CAD build for the part. Positions are in the model's coordinates, mm. Face numbers are marked on the shaded views. A direction names the side the tool comes from. Give positions to 0.01 mm unless a question says otherwise; leave off trailing zeros. Write each loop counter-clockwise with the first axis right and the second up, starting at its lowest first coordinate (ties: lowest second). Pieces come first, ordered by that corner, then holes. Notation, with made-up numbers: (-2.5, -17) - (11.5, -17) arc R31 cw to (11.5, 18) - close; hole circle Ø7 at (-26.5, 53.25). An arc over 180 degrees is marked (long way). Answer as a JSON object with one key per item and string values.
from build123d import *

# Parameters (mm, degrees)
CROQUIS1_W              = 202
CROQUIS1_H              = 100
SALIENTE_EXTRUIR1_DEPTH = 1.5
CROQUIS2_R              = 1.6
CORTAR_EXTRUIR1_DEPTH   = 1.5
CROQUIS3_W              = 12
CROQUIS3_H              = 100
CROQUIS3_R              = 1.6
SALIENTE_EXTRUIR2_DEPTH = 6
CROQUIS4_W              = 47
CROQUIS4_H              = 28
CROQUIS4_W_2            = 76
SALIENTE_EXTRUIR3_DEPTH = 1.5
REDONDEO1_R             = 10
REDONDEO2_R             = 10
CROQUIS5_R              = 3
CORTAR_EXTRUIR2_DEPTH   = 2


with BuildPart() as part:
    # Croquis1 → Saliente-Extruir1 (new body)
    with BuildSketch(Plane(origin=(0, 0, 0), x_dir=(1, 0, 0), z_dir=(0, 1, 0))):
        with Locations((101, 50)):
            Rectangle(CROQUIS1_W, CROQUIS1_H)
    extrude(amount=SALIENTE_EXTRUIR1_DEPTH)

    # Croquis2 → Cortar-Extruir1 (cut)
    with BuildSketch(Plane(origin=(0, 1.5, 0), x_dir=(1, 0, 0), z_dir=(0, 1, 0))):
        with Locations(Location((6, 85, 0), (0, 0, 270))):
            Circle(CROQUIS2_R)
        with Locations(Location((6, 15, 0), (0, 0, 270))):
            Circle(CROQUIS2_R)
    extrude(amount=-CORTAR_EXTRUIR1_DEPTH, mode=Mode.SUBTRACT)

    # Croquis3 → Saliente-Extruir2 (add)
    with BuildSketch(Plane.XZ):
        with Locations((6, -50)):
            Rectangle(CROQUIS3_W, CROQUIS3_H)
        with Locations(Location((6, -15, 0), (0, 0, 90))):
            Circle(CROQUIS3_R, mode=Mode.SUBTRACT)
        with Locations(Location((6, -85, 0), (0, 0, 90))):
            Circle(CROQUIS3_R, mode=Mode.SUBTRACT)
    extrude(amount=SALIENTE_EXTRUIR2_DEPTH)

    # Croquis4 → Saliente-Extruir3 (add)
    with BuildSketch(Plane(origin=(0, 1.5, 0), x_dir=(1, 0, 0), z_dir=(0, 1, 0))):
        with Locations((61.5, -14)):
            Rectangle(CROQUIS4_W, CROQUIS4_H)
        with Locations((164, -14)):
            Rectangle(CROQUIS4_W_2, CROQUIS4_H)
    extrude(amount=-SALIENTE_EXTRUIR3_DEPTH)

    # Redondeo1
    redondeo1_edges = [part.edges().sort_by_distance(p)[0] for p in [
        (85, 0.75, 0),
        (38, 0.75, 0),
        (126, 0.75, 0),
    ]]
    fillet(redondeo1_edges, radius=REDONDEO1_R)

    # Redondeo2
    # the kernel refuses this fillet: 10 mm, written as the material it adds along each edge
    with BuildSketch(Plane(origin=(12, 0, -100), x_dir=(0, -1, 0), z_dir=(0, 0, 1))) as redondeo2_piece_1:
        with BuildLine():
            CenterArc((10, 9.16515139), REDONDEO2_R, 180, 66.421821522)
            Line((0, 9.16515139), (-0.2, 9.16515139))
            Line((-0.2, 9.16515139), (-0.2, 0))
            Line((-0.2, 0), (0, -0.2))
            ThreePointArc((0, -0.2), (3, -0.2), (5.92, -0.183303028))
            Line((5.92, -0.183303028), (6, 0))
        make_face()
    extrude(amount=100)

    # Croquis5 → Cortar-Extruir2 (cut)
    with BuildSketch(Plane(origin=(0, 1.5, 0), x_dir=(1, 0, 0), z_dir=(0, 1, 0))):
        with Locations(Location((6, 85, 0), (0, 0, 270))):
            Circle(CROQUIS5_R)
        with Locations(Location((6, 15, 0), (0, 0, 270))):
            Circle(CROQUIS5_R)
    extrude(amount=-CORTAR_EXTRUIR2_DEPTH, mode=Mode.SUBTRACT)


solid = part.part
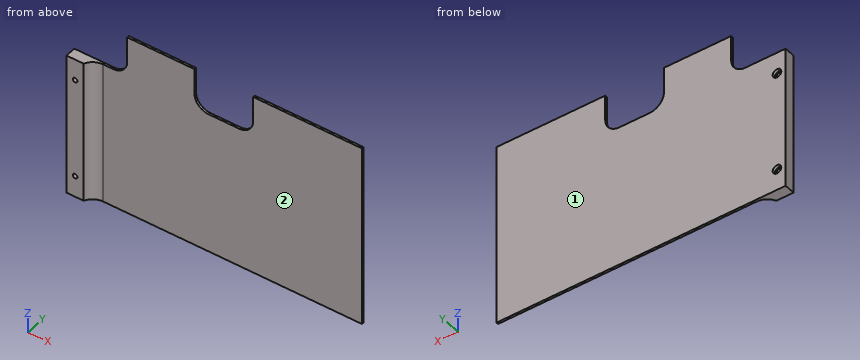
Item 1: Probe line 1 (X direction, y = 0.1, z = -15); line 2 (Z direction, x = 6, y = -3.95); line 3 (Z direction, x = 14, y = -1). List the from-to ranges inside material, lowest first. Write a range as from..to.
Entries:
{"line 1": "0..3, 9..202", "line 2": "-100..-86.6, -83.4..-16.6, -13.4..0", "line 3": "-100..0"}
Item 2: Cut at A-A (z = -79.5). Give the cut face in (x, y).
Entries:
{"outline": "(0, -6) - (12, -6) arc R10 cw to (21.17, 0) - (202, 0) - (202, 1.5) - (0, 1.5) - close"}
Item 3: Flat gauge pins, fed straight in: P1, Ø1.2, axis at y = 1, z = 23.5, coming from the -X side; P2, Ø3, axis at x = 6, z = -15, coming from the +Y side; P3, Ø1.5, axis at y = -5, z = -11.5, coming from the +X side; P4, Ø1.8, axis at x = 5, z = -15.5, coming from the +Y side. Where does each tip first touch, or does it go through?
Entries:
{"P1": "x = 38", "P2": "through", "P3": "x = 12.98", "P4": "y = -0.5"}
Item 4: Cut at C-C (y = -3.75). Give the cut face in (x, z), and give its area (3 significant figures).
Entries:
{"outline": "(0, -100) - (13.36, -100) - (13.36, 0) - (0, 0) - close; hole circle Ø3.2 at (6, -85); hole circle Ø3.2 at (6, -15)", "area": "1,320 mm2"}
Item 5: Which spindle directions (+Z, -Z, +X, -X, +Y, -Y) get a long thin tool onto all of the face, cutting with end or side? Do the marked faces 1 and 2. Say none if no direction does.
Entries:
{"face 1": "+Z, -Z, +X, -X, +Y", "face 2": "+Z, -Z, +X, -Y"}
Item 6: Cut at B-B (x = 74). Give the cut face in (y, z), and give its area (3 significant figures).
Entries:
{"outline": "(0, -100) - (1.5, -100) - (1.5, 28) - (0, 28) - close", "area": "192 mm2"}
